Read the model definition and answer for the solid it produces. Units are mm, in the model's axes. Face numbers are marked on the shaded views. A direction names the side the tool comes from. Give positions to 0.01 mm unless a question says otherwise; leave off trailing zeros. Order: outer loops, then holes, each group sorted by start corner. A loop starts at its lowest first (then second) coordinate and runs counter-clockwise, first axis right, second up.
Item 1: Find the intervals of material crossed by line 1 along Z through (x, y) = (4.5, 3.75); line 2 along Y through (x, z) = (10.5, 14); line 3 along Z through (x, y) = (15.5, 5.75), in increasing order.
Item 2: Which of the six approach directions +Z, -Z, +X, -X, +Y, -Y give full straight-line access (tool end or side, diameter ignored) to the marked faces 1, 2 and 3?
Item 3: A cutting plane is placed at A-A (x = 17.5). Write down the section's boundary in (y, z).
Item 4: Given pin 1 Ø3.5 at (x, y) = (15, 3.5) entering from +Z; pin 2 Ø6 at (y, z) = (2, 27) entering from +X; pin 3 Ø3 at (y, z) = (4, 27) entering from -X, each flat-ended and moving along its own axis, determine where each tip first touches the part or whether it passes through.
Item 5: A cutting plane is placed at D-D (x = 4). Write down the section's boundary in (y, z), plus the area to 3 significant figures.
Item 6: A cutting plane is placed at B-B (y = 9). Write down the section's boundary in (x, z), plus the area to 3 significant figures.
Item 7: A cutting plane is placed at C-C (z = 19). Write down the section's boundary in (x, y).
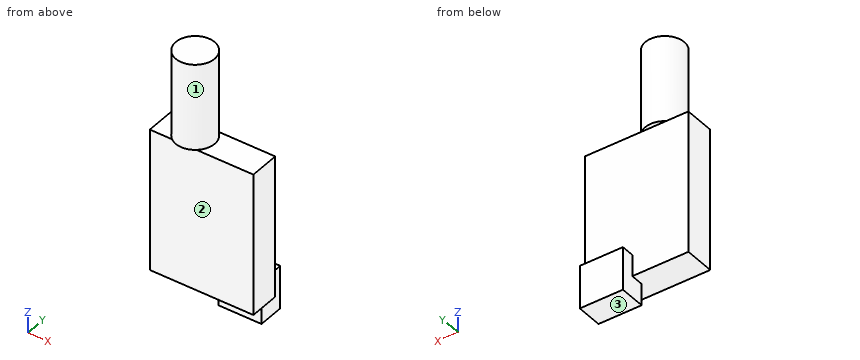
from build123d import *

# Parameters (mm, degrees)
F0_W     = 10
F0_H     = 5
F1_DEPTH = 7
F2_DEPTH = 3
F3_R     = 4.5
F4_DEPTH = 20
F5_ANGLE = 180


with BuildPart() as f1:
    # F0 (on Front) → F1 (new body)
    with BuildSketch(Plane.XZ):
        Polygon((12, -16.5), (12, 16.5), (-12, 16.5), (-12, -16.5), (-11, -16.5), (-11, -11.5), (-1, -11.5), (-1, -16.5), align=None)
        with Locations((-6, -14)):
            Rectangle(F0_W, F0_H)
    extrude(amount=-F1_DEPTH)

    # F0 (on Front) → F2 (join, symmetric)
    with BuildSketch(Plane.XZ):
        with Locations((-6, -19)):
            Rectangle(F0_W, F0_H)
        with Locations((-6, -14)):
            Rectangle(F0_W, F0_H)
    extrude(amount=F2_DEPTH, both=True)

    # F3 (on face) → F4 (join)
    with BuildSketch(Plane.XY.offset(16.5)):
        with Locations((4, 3.5)):
            Circle(F3_R)
    extrude(amount=F4_DEPTH)


with BuildPart() as f1_1:
    # F5: moved
    add(f1.part.rotate(Axis((4, 3.5, 16.5), (0, 0, -1)), F5_ANGLE))


solid = f1_1.part
Response values:
1. line 1: z = -16.5 to 36.5
1. line 2: y = 0 to 7
1. line 3: z = -21.5 to 16.5
2. face 1: +Z
2. face 2: -Z, +X, -X, -Y
2. face 3: -Z, +X, -X, +Y, -Y
3. outline: (0, -16.5) - (4, -16.5) - (4, -21.5) - (10, -21.5) - (10, -11.5) - (7, -11.5) - (7, 16.5) - (0, 16.5) - close
4. pin 1: stops at z = 16.5
4. pin 2: stops at x = 8.5
4. pin 3: stops at x = -0.5
5. outline: (-1, 16.5) - (0, 16.5) - (0, -16.5) - (7, -16.5) - (7, 16.5) - (8, 16.5) - (8, 36.5) - (-1, 36.5) - close
5. area: 411 mm2
6. outline: (9, -21.5) - (19, -21.5) - (19, -11.5) - (9, -11.5) - close
6. area: 100 mm2
7. outline: circle Ø9 at (4, 3.5)
